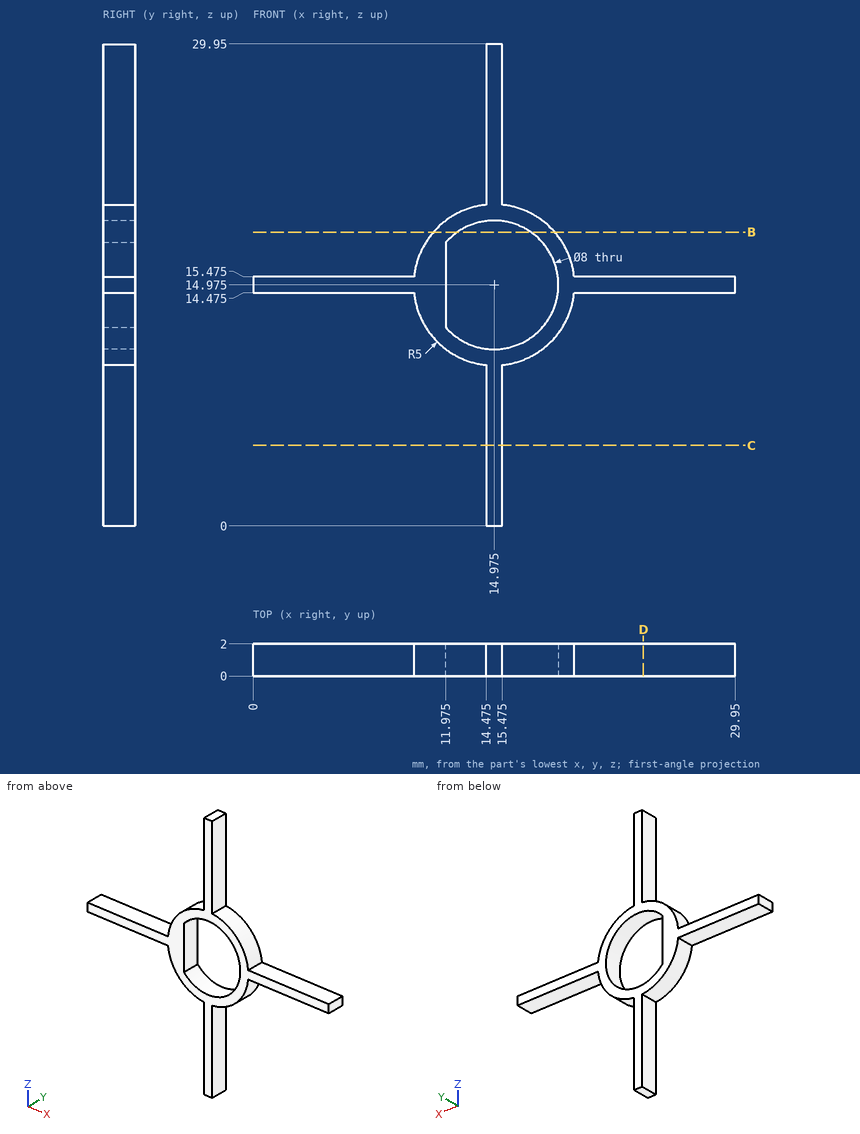
Verification items for this drawing (mm, ordinates from the low corner). Coordinates: 2 decimals unless noted, no trailing zeros. Write each loop counter-clockwise with the first axis right and the second up, starting at its lowest first coordinate (ties: lowest second). Pieces come first, ordered by that corner, then holes. Notation, with made-up numbers: M 41,11.25 L 87,11.25 A10 cw 87,22.25 Z; hole C 86.25,-10 d9. An arc over 180 degrees is marked long. Use CSV: the item, a comma, the result in double quotes.
Q1. Section check D-D, the plane x = 24.25. Enter the section's corners in (y, z) (3 decimals).
Computed values:
outline,"M 0,14.475 L 2,14.475 L 2,15.475 L 0,15.475 Z"
Q2. Section check B-B, the plane z = 18.25. Enter the section's corners in (x, y).
Computed values:
outline,"M 11.2,0 L 12.68,0 L 12.68,2 L 11.2,2 Z; M 17.27,0 L 18.75,0 L 18.75,2 L 17.27,2 Z"
Q3. Thickness scan on line 1 along Z through (x, y) = (15, 0.45) (3 decimals); line 2 along Z through (x, y) = (4.5, 0.65) (3 decimals). Record the ranges inside material, lowest first. Write a range as [from, to].
Computed values:
line 1,"[0, 10.975], [18.975, 29.95]"
line 2,"[14.475, 15.475]"
Q4. Section check C-C, the plane z = 5. Enter the section's corners in (x, y) (3 decimals), and give its area (3 significant figures).
Computed values:
outline,"M 14.475,0 L 15.475,0 L 15.475,2 L 14.475,2 Z"
area,"2.00 mm²"
Q5. Go/stop test with flat-tipped pins: P1, Ø1, axis at y = 1, z = 25.5, coming from the +X side (3 decimals); P2, Ø0.6, axis at x = 24, y = 1.5, coming from the +Z side (3 decimals); P3, Ø1, axis at x = 4, y = 1, coming from the -Z side (3 decimals). Record where each tip stops, or that it passes through.
Computed values:
P1,"x = 15.475"
P2,"z = 15.475"
P3,"z = 14.475"
